Here's how the part is built. I have some questions about the finished solid (model axes, mm). Face numbers are marked on the shaded views. A direction names the side the tool comes from. Round coordinates to 2 decimals unless told otherwise and drop trailing zeros. Write each loop counter-clockwise with the first axis right and the second up, starting at its lowest first coordinate (ties: lowest second). Pieces come first, ordered by that corner, then holes. Notation, with made-up numbers: (-28.75, -3.5) -> (-8.75, -3.5) arc R26 cw to (-8.75, 18.5) -> close; hole circle Ø9 at (-6.5, 51). An arc over 180 degrees is marked (long way). Answer as CSV lines item,"result".
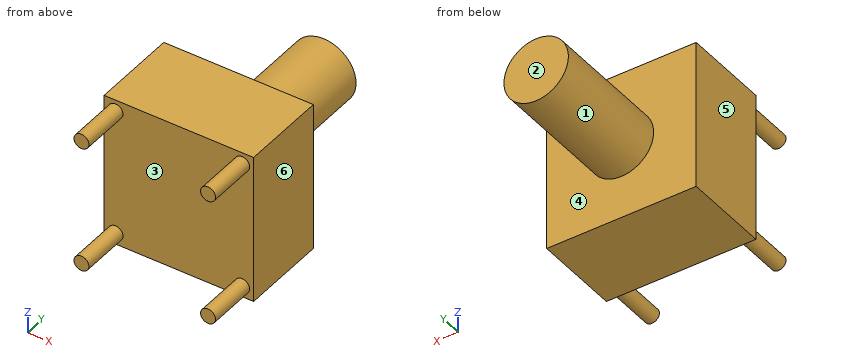
from build123d import *

# Parameters (mm, degrees)
SKETCH1_W           = 6
SKETCH1_H           = 6
BOSS_EXTRUDE1_DEPTH = 3.5
SKETCH2_R           = 1.292115179
BOSS_EXTRUDE2_DEPTH = 5
SKETCH3_R           = 0.3
BOSS_EXTRUDE3_DEPTH = 2


with BuildPart() as part:
    # Sketch1 → Boss-Extrude1 (new body)
    with BuildSketch(Plane(origin=(0, 0, 0), x_dir=(1, 0, 0), z_dir=(0, 1, 0))):
        with Locations((3, 3)):
            Rectangle(SKETCH1_W, SKETCH1_H)
    extrude(amount=BOSS_EXTRUDE1_DEPTH)

    # Sketch2 → Boss-Extrude2 (add)
    with BuildSketch(Plane(origin=(0, 3.5, 0), x_dir=(1, 0, 0), z_dir=(0, 1, 0))):
        with Locations((2.999291, 3)):
            Circle(SKETCH2_R)
    extrude(amount=BOSS_EXTRUDE2_DEPTH)

    # Sketch3 → Boss-Extrude3 (add)
    with BuildSketch(Plane(origin=(0, 0, 0), x_dir=(-1, 0, 0), z_dir=(0, -1, 0))):
        with Locations((-0.46, 0.46)):
            Circle(SKETCH3_R)
        with Locations((-5.54, 0.46)):
            Circle(SKETCH3_R)
        with Locations((-0.46, 5.54)):
            Circle(SKETCH3_R)
        with Locations((-5.54, 5.548881257)):
            Circle(SKETCH3_R)
    extrude(amount=BOSS_EXTRUDE3_DEPTH)


solid = part.part
Item 1: Suppose I cut it at B-B, the plane x = 3. List the corners of the cut face in (y, z) for me, then the cut area to 3 significant figures.
Results found:
outline,"(0, -6) -> (3.5, -6) -> (3.5, -4.29) -> (8.5, -4.29) -> (8.5, -1.71) -> (3.5, -1.71) -> (3.5, 0) -> (0, 0) -> close"
area,"33.9 mm²"
Item 2: Suppose I cut it at A-A, the plane z = -0.46. List the corners of the cut face in (x, y) for me.
Results found:
outline,"(0, 0) -> (0.16, 0) -> (0.16, -2) -> (0.76, -2) -> (0.76, 0) -> (5.24, 0) -> (5.24, -2) -> (5.84, -2) -> (5.84, 0) -> (6, 0) -> (6, 3.5) -> (0, 3.5) -> close"
Item 3: Suppose I cut it at C-C, the plane y = -0.75. List the corners of the cut face in (x, z) for me.
Results found:
outline,"circle Ø0.6 at (0.46, -5.54); circle Ø0.6 at (0.46, -0.46); circle Ø0.6 at (5.54, -5.55); circle Ø0.6 at (5.54, -0.46)"
Item 4: For the marked faces 1 and 2, which set-ups out of +Z, -Z, +X, -X, +Y, -Y let a thin tool reach every point of the face, with its end or its side?
Results found:
face 1,"+Y"
face 2,"+Z, -Z, +X, -X, +Y"
Item 5: If we mould it in two halves opening along X, with no side actions, what happens to the marked faces 3, 4, 5 and 6? For each: pulls with the +X half, pulls with the -X half, needs draft (parallel to the pull), parting line crosses it, or undercut.
Results found:
face 3,"undercut"
face 4,"needs draft"
face 5,"pulls with the -X half"
face 6,"pulls with the +X half"
Item 6: I need wall thicknesses on L1, parallel to Y at x = 2.3, z = -4.9; L2, parallel to Y at x = 2.4, z = -4.1; L3, parallel to X at y = 4.25, z = -3.1. Which ranges of each line are inside material? Lowest first, please.
Results found:
L1,"y = 0 to 3.5"
L2,"y = 0 to 8.5"
L3,"x = 1.71 to 4.29"
Item 7: Suppose I cut it at D-D, the plane z = -3. List the corners of the cut face in (x, y) for me, then the cut area to 3 significant figures.
Results found:
outline,"(0, 0) -> (6, 0) -> (6, 3.5) -> (4.29, 3.5) -> (4.29, 8.5) -> (1.71, 8.5) -> (1.71, 3.5) -> (0, 3.5) -> close"
area,"33.9 mm²"
Item 8: Will this pin go through, and if not, where does the flat tip stop? pin 1 (3 mm diameter, centred on x = 2.5, z = -2.5, fed in from -Y).
Results found:
pin 1,"stops at y = 0"
